Job drawing, mm, ordinate dimensions from the low corner. One solid piece. A direction names the side the tool comes from. Coordinates: 2 decimals unless noted, no trailing zeros. Write each loop counter-clockwise with the first axis right and the second up, starting at its lowest first coordinate (ties: lowest second). Pieces come first, ordered by that corner, then holes. Notation, with made-up numbers: (65, 48) - (122, 48) arc R10 ccw to (122, 57) - close; hole circle Ø4 at (36, 80). An arc over 180 degrees is marked (long way). Use a Markdown table: item, result.
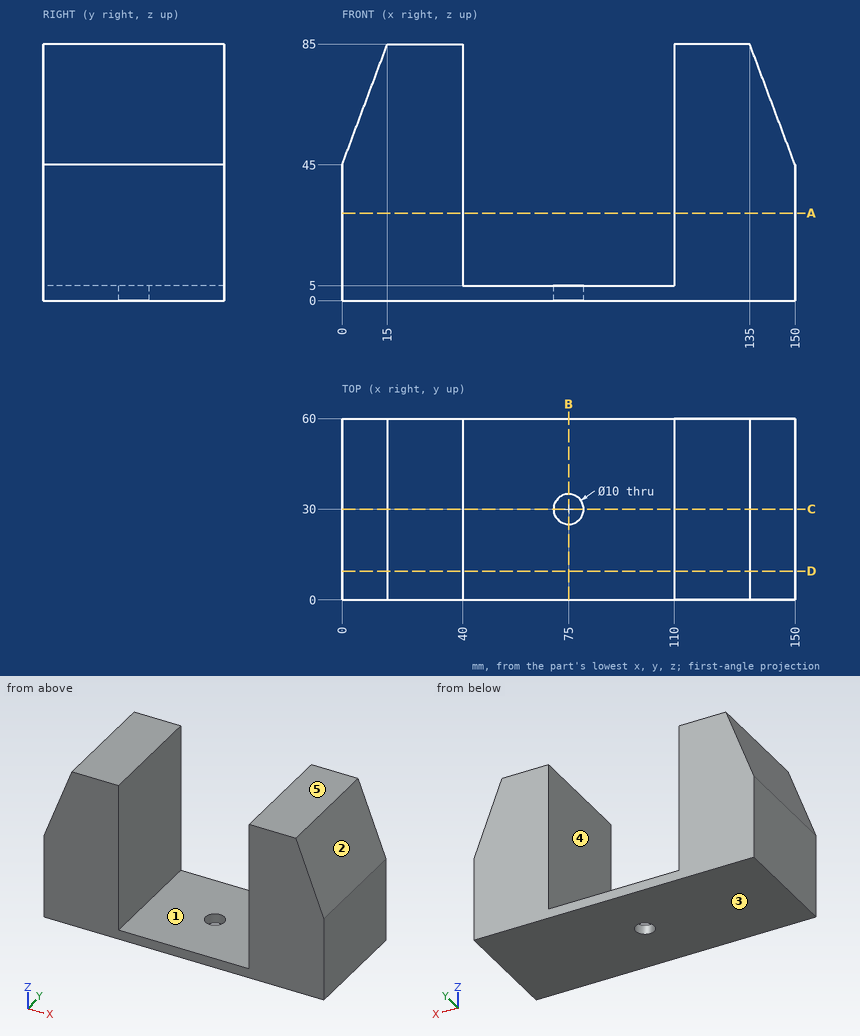
Item 1: Band-saw the part on C-C, the plane y = 30. Give the cut face in (x, z).
From the geometry:
| item | result |
|---|---|
| outline | (0, 0) - (70, 0) - (70, 5) - (40, 5) - (40, 85) - (15, 85) - (0, 45) - close; (80, 0) - (150, 0) - (150, 45) - (135, 85) - (110, 85) - (110, 5) - (80, 5) - close |
Item 2: Which spindle directions (+Z, -Z, +X, -X, +Y, -Y) get a long thin tool onto all of the face, cutting with end or side? Do the marked faces 4 and 5. Say none if no direction does.
From the geometry:
| item | result |
|---|---|
| face 4 | +Z, +Y, -Y |
| face 5 | +Z, +X, -X, +Y, -Y |
Item 3: Band-saw the part on A-A, the plane z = 29. Give the cut face in (x, y), then the cut area to 3 significant figures.
From the geometry:
| item | result |
|---|---|
| outline | (0, 0) - (40, 0) - (40, 60) - (0, 60) - close; (110, 0) - (150, 0) - (150, 60) - (110, 60) - close |
| area | 4,800 mm^2 |
Item 4: Drop flat-ended pins along their axis: P1, Ø2, axis at x = 80.5, y = 25.5, coming from the -Z side; P2, Ø6, axis at y = 19.5, z = 68.5, coming from the +X side; P3, Ø13, axis at x = 75, y = 30, coming from the +Z side; P4, Ø6, axis at y = 49, z = 70, coming from the +X side. Give the stop position or say it passes through.
From the geometry:
| item | result |
|---|---|
| P1 | z = 0 |
| P2 | x = 142.31 |
| P3 | z = 5 |
| P4 | x = 141.75 |
Item 5: Two-plate mould, pull along X, no slides. Class the marked faces 1, 2 and 3: pulls with the +X half, pulls with the -X half, needs draft (parallel to the pull), parting line crosses it, or undercut.
From the geometry:
| item | result |
|---|---|
| face 1 | undercut |
| face 2 | pulls with the +X half |
| face 3 | needs draft |
Item 6: Band-saw the part on B-B, the plane x = 75. Give the cut face in (y, z).
From the geometry:
| item | result |
|---|---|
| outline | (0, 0) - (25, 0) - (25, 5) - (0, 5) - close; (35, 0) - (60, 0) - (60, 5) - (35, 5) - close |
Item 7: Band-saw the part on D-D, the plane y = 9.5. Give the cut face in (x, z).
From the geometry:
| item | result |
|---|---|
| outline | (0, 0) - (150, 0) - (150, 45) - (135, 85) - (110, 85) - (110, 5) - (40, 5) - (40, 85) - (15, 85) - (0, 45) - close |
Item 8: Drill centre lines: probe 1 along Y at (x, z) = (75, 2.75); probe 2 along X at (y, z) = (15, 42); probe 3 along Z at (x, y) = (72.5, 44). Where is each one in solid material? Low to high.
From the geometry:
| item | result |
|---|---|
| probe 1 | 0 to 25, 35 to 60 |
| probe 2 | 0 to 40, 110 to 150 |
| probe 3 | 0 to 5 |
